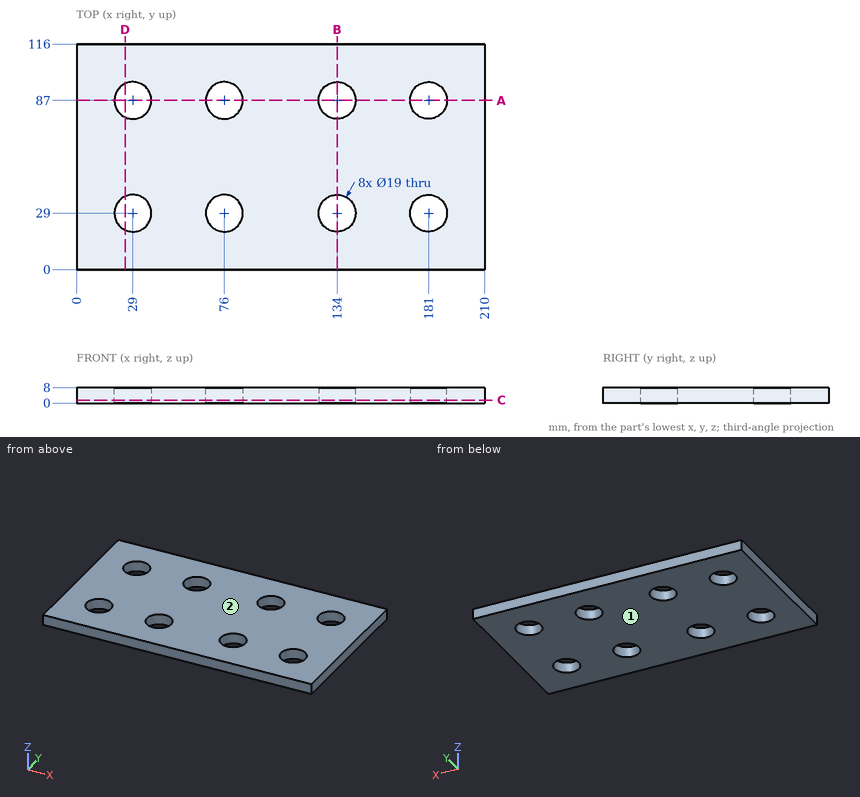
Design review of the part shown in the three views and the two pictorial views. Dimensions are in mm from the part's minimum x, y and z. Give positions to 0.01 mm unless a question says otherwise; leave off trailing zeros. Loops run counter-clockwise (first coordinate to the right, second up) from the corner with the lowest first, then second, coordinate; pieces in that order, holes last. Notation, with made-up numbers: (-3.75, -3.75) -> (23.25, -3.75) arc R33 ccw to (23.25, 26.25) -> close; hole circle Ø5 at (8.5, 38). An arc over 180 degrees is marked (long way). Write each question's results on one line, items separated by ' | '.
1) For line 1 along Y through (x, z) = (181, 2); line 2 along X through (y, z) = (22, 6.5); line 3 along Y through (x, z) = (127, 6.5), list the stretches that pass through material, from the lowest coordinate up. Write a range as from..to.
Conclusion:
line 1: y = 0..19.5, 38.5..77.5, 96.5..116 | line 2: x = 0..22.58, 35.42..69.58, 82.42..127.58, 140.42..174.58, 187.42..210 | line 3: y = 0..22.58, 35.42..80.58, 93.42..116
2) Take a section at A-A, the plane y = 87. Give the boundary of the cut face in (x, z), plus the area to 3 significant figures.
Conclusion:
outline: (0, 0) -> (19.5, 0) -> (19.5, 8) -> (0, 8) -> close; (38.5, 0) -> (66.5, 0) -> (66.5, 8) -> (38.5, 8) -> close; (85.5, 0) -> (124.5, 0) -> (124.5, 8) -> (85.5, 8) -> close; (143.5, 0) -> (171.5, 0) -> (171.5, 8) -> (143.5, 8) -> close; (190.5, 0) -> (210, 0) -> (210, 8) -> (190.5, 8) -> close | area: 1,070 mm^2
3) Take a section at D-D, the plane x = 25. Give the boundary of the cut face in (y, z), plus the area to 3 significant figures.
Conclusion:
outline: (0, 0) -> (20.38, 0) -> (20.38, 8) -> (0, 8) -> close; (37.62, 0) -> (78.38, 0) -> (78.38, 8) -> (37.62, 8) -> close; (95.62, 0) -> (116, 0) -> (116, 8) -> (95.62, 8) -> close | area: 652 mm^2
4) Take a section at C-C, the plane z = 1.5. Count the separate pieces of the cut face and the enclosed holes in it, plus the area to 3 significant figures.
Conclusion:
separate pieces: 1 | enclosed holes: 8 | area: 22,100 mm^2
5) Take a section at B-B, the plane x = 134. Give the boundary of the cut face in (y, z), plus the area to 3 significant figures.
Conclusion:
outline: (0, 0) -> (19.5, 0) -> (19.5, 8) -> (0, 8) -> close; (38.5, 0) -> (77.5, 0) -> (77.5, 8) -> (38.5, 8) -> close; (96.5, 0) -> (116, 0) -> (116, 8) -> (96.5, 8) -> close | area: 624 mm^2
6) Draft analysis for pull direction Z (two halves, no side actions). For the marked faces 1 and 2, state which applies: pulls with the +Z half, pulls with the -Z half, needs draft (parallel to the pull), parting line crosses it, or undercut.
Conclusion:
face 1: pulls with the -Z half | face 2: pulls with the +Z half
